from build123d import *

# Parameters (mm, degrees)
SKETCH1_R               = 28.334624745
BOSS_EXTRUDE1_DEPTH     = 4.5
CUT_EXTRUDE2_DEPTH      = 5.5
CIRPATTERN1_COUNT       = 17
CUT_EXTRUDE4_DEPTH      = 6.5
CUT_EXTRUDE4_DEPTH_BACK = 6.5
SKETCH3_R               = 4.7625


with BuildPart() as part:
    # Sketch1 → Boss-Extrude1 (new body)
    with BuildSketch(Plane.XY):
        Circle(SKETCH1_R)
    extrude(amount=BOSS_EXTRUDE1_DEPTH)

    # Sketch2 → Cut-Extrude2 (cut, symmetric)
    with BuildSketch(Plane.XY):
        Polygon((23.37843536, -2.54), (29.534624745, -4), (29.534624745, 4), (23.37843536, 2.54), align=None)
    cut_extrude2 = extrude(amount=CUT_EXTRUDE2_DEPTH, both=True, mode=Mode.SUBTRACT)

    # CirPattern1: Cut-Extrude2 ×17 about axis
    cirpattern1_axis = Axis((0, 0, 0), (0, 0, 1))
    for i in range(1, CIRPATTERN1_COUNT):
        add(cut_extrude2.rotate(cirpattern1_axis, i * 360 / CIRPATTERN1_COUNT), mode=Mode.SUBTRACT)

    # Sketch3 → Cut-Extrude4 (cut, two sides: drawn at the far end of the back side and taken through both)
    with BuildSketch(Plane.XY.offset(-CUT_EXTRUDE4_DEPTH_BACK)):
        with Locations(Location((0, 0, 0), (0, 0, 180))):
            Circle(SKETCH3_R)
    extrude(amount=CUT_EXTRUDE4_DEPTH + CUT_EXTRUDE4_DEPTH_BACK, mode=Mode.SUBTRACT)


solid = part.part
Check sheet for the modelled part. Datum: model origin and axes. Units: mm. A direction names the side the tool comes from. Round coordinates to 2 decimals unless told otherwise and drop trailing zeros. Loops run counter-clockwise (first coordinate to the right, second up) from the corner with the lowest first, then second, coordinate; pieces in that order, holes last.
1. Sectioned sample at C-C on y = -9.5. Record the boundary of the cut face in (x, z).
2. Scan lines: probe 1 along Y at (x, z) = (-13, 4.2); probe 2 along Y at (x, z) = (25, 1.8); probe 3 along Y at (x, z) = (0, 1). Record each from-to range of solid material in increasing order.
3. Set-up check for faces 5 (the flat face through (-0.716, 25.948, 2.282)), 6 (the flat face through (-0.707, -25.88, 2.282)), 7 (the flat face through (-24.76, -7.79, 2.28)), 8 (the flat face through (-4.064, -25.638, 2.282)), 9 (the flat face through (22.9, 12.2, 2.3)): record each of +Z, -Z, +X, -X, +Y, -Y from which the full face is reachable in a straight line by a thin tool's end or side.
4. Gauge pin test, flat ends, axial feed: pin 1 Ø1.3 at (y, z) = (1, 2.5) entering from +X; pin 2 Ø1.5 at (x, z) = (6, 0.5) entering from +Y; pin 3 Ø10 at (x, y) = (4.5, 8.5) entering from -Z; pin 4 Ø1.5 at (x, z) = (3, 1) entering from +Y. Record the tip position at first contact, or that the pin passes through.
5. Sectioned sample at B-B on x = 1. Record the boundary of the cut face in (y, z).
6. Mould release check, pull along Y, two halves, no side actions. Record for faces 1 (the flat face through (-7, 0, 0)), 2 (the flat face through (21.813, -8.412, 2.282)), 3 (the flat face through (-14.06, -18.68, 2.28)), 4 (the flat face through (2.122, 23.282, 2.282)): released by +Y, released by -Y, zero draft, split by the parting line, or undercut.
7. Sectioned sample at A-A on y = 0. Record the boundary of the cut face in (x, z), and give its area (3 significant figures).
Recorded:
1. outline: (-26.69, 0) - (21.39, 0) - (21.39, 4.5) - (-26.69, 4.5) - close
2. probe 1: y = -25.18 to -22.32, -19.48 to 19.48, 22.32 to 25.18
2. probe 2: y = -6.39 to -2.92, 2.92 to 6.39
2. probe 3: y = -23.48 to -4.76, 4.76 to 23.48
3. face 5: +Z, -Z, +Y
3. face 6: +Z, -Z, -Y
3. face 7: +Z, -Z, -X
3. face 8: +Z, -Z
3. face 9: +Z, -Z, +X
4. pin 1: stops at x = 23.38
4. pin 2: stops at y = 27.64
4. pin 3: stops at z = 0
4. pin 4: stops at y = 23.27
5. outline: (-23.39, 0) - (-4.66, 0) - (-4.66, 4.5) - (-23.39, 4.5) - close; (4.66, 0) - (23.39, 0) - (23.39, 4.5) - (4.66, 4.5) - close
6. face 1: zero draft
6. face 2: undercut
6. face 3: undercut
6. face 4: released by +Y
7. outline: (-28.33, 0) - (-4.76, 0) - (-4.76, 4.5) - (-28.33, 4.5) - close; (4.76, 0) - (23.38, 0) - (23.38, 4.5) - (4.76, 4.5) - close
7. area: 190 mm2
